from build123d import *

# Parameters (mm, degrees)
EXTRUDE_1_DEPTH     = 20
SKETCH_2_W          = 18
SKETCH_2_H          = 16
CUT_EXTRUDE_1_DEPTH = 18
SKETCH_3_R          = 1.75
CUT_EXTRUDE_2_DEPTH = 18
SKETCH_4_R          = 1.75
CUT_EXTRUDE_3_DEPTH = 18


with BuildPart() as part:
    # 草图1 → 凸台-拉伸1 (new body)
    with BuildSketch(Plane.XY):
        Polygon((2, 20), (20, 2), (20, 0), (0, 0), (0, 20), align=None)
    extrude(amount=EXTRUDE_1_DEPTH)

    # 草图2 → 切除-拉伸1 (cut)
    with BuildSketch(Plane(origin=(0, 20, 0), x_dir=(1, 0, 0), z_dir=(0, 1, 0))):
        with Locations((11, -10)):
            Rectangle(SKETCH_2_W, SKETCH_2_H)
    extrude(amount=-CUT_EXTRUDE_1_DEPTH, mode=Mode.SUBTRACT)

    # 草图3 → 切除-拉伸2 (cut)
    with BuildSketch(Plane.XZ):
        with Locations(Location((10, 10, 0), (0, 0, 270))):
            Circle(SKETCH_3_R)
    extrude(amount=-CUT_EXTRUDE_2_DEPTH, mode=Mode.SUBTRACT)

    # 草图4 → 切除-拉伸3 (cut)
    with BuildSketch(Plane.ZY):
        with Locations((10, 10)):
            Circle(SKETCH_4_R)
    extrude(amount=-CUT_EXTRUDE_3_DEPTH, mode=Mode.SUBTRACT)


solid = part.part
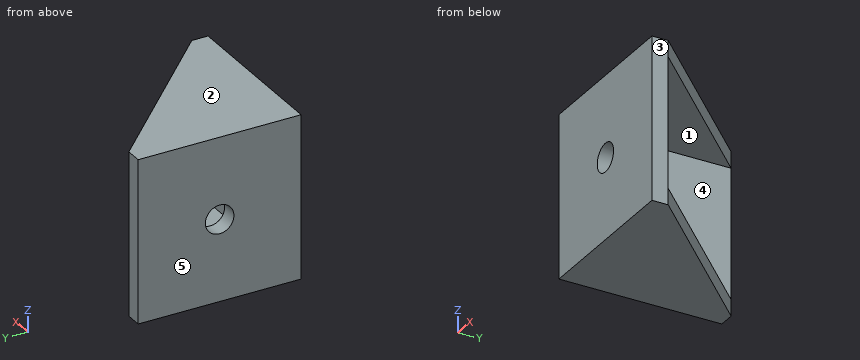
Here's how the part is built. I have some questions about the finished solid (model axes, mm). Face numbers are marked on the shaded views. A direction names the side the tool comes from. Coordinates: 2 decimals unless noted, no trailing zeros. Write each loop counter-clockwise with the first axis right and the second up, starting at its lowest first coordinate (ties: lowest second). Pieces come first, ordered by that corner, then holes.
Item 1: If we mould it in two halves opening along Z, with no side actions, what happens to the marked faces 1, 2 and 3? For each: +Z half, -Z half, draft (parallel to the pull), parting line (faces both ways), or undercut.
Item 2: I want a section at C-C on z = 10. Write out the boundary of the cut face in (x, y), and give its area (3 significant figures).
Item 3: I want a section at A-A on x = 10. Write out the boundary of the cut face in (y, z), and give its area (3 significant figures).
Item 4: I want a section at D-D on x = 1.5. Write out the boundary of the cut face in (y, z).
Item 5: Will these pins go through, and if not, where does the flat tip stop? pin 1 (5.5 mm diameter, centred on y = 10, z = 10, fed in from +X); pin 2 (8 mm diameter, centred on x = 10.5, z = 9, fed in from +Y).
Item 6: On a 3-axis mill with a long thin cutter (end or side, diameter ignored), from which of +Z, -Z, +X, -X, +Y, -Y can I reach the whole of each face in a straight line? I mean the marked faces 4 and 5. Say none if no direction works.
Item 7: If I drill on line 1 (X direction, y = 0.8, z = 10); line 2 (Z direction, x = 9.75, y = 8.5); line 3 (X direction, y = 6.75, z = 6), over which ranges is the centre line in solid material (lowest first)?
Findings below:
1. face 1: undercut
1. face 2: +Z half
1. face 3: draft
2. outline: (0, 0) - (8.25, 0) - (8.25, 2) - (2, 2) - (2, 8.25) - (0, 8.25) - close; (0, 11.75) - (2, 11.75) - (2, 20) - (0, 20) - close; (11.75, 0) - (20, 0) - (20, 2) - (11.75, 2) - close
2. area: 62.0 mm2
3. outline: (0, 0) - (12, 0) - (12, 2) - (2, 2) - (2, 8.25) - (0, 8.25) - close; (0, 11.75) - (2, 11.75) - (2, 18) - (12, 18) - (12, 20) - (0, 20) - close
3. area: 73.0 mm2
4. outline: (0, 0) - (20, 0) - (20, 20) - (0, 20) - close; hole circle Ø3.5 at (10, 10)
5. pin 1: stops at x = 2
5. pin 2: stops at y = 2
6. face 4: +X, +Y
6. face 5: +Z, -Z, -X, +Y, -Y
7. line 1: x = 0 to 8.25, 11.75 to 20
7. line 2: z = 0 to 2, 18 to 20
7. line 3: x = 0 to 2
